Design review of the part built by this model. Coordinates are the model's own, in mm. A direction names the side the tool comes from. Give positions to 0.01 mm unless a question says otherwise; leave off trailing zeros. Order: outer loops, then holes, each group sorted by start corner. A loop starts at its lowest first (then second) coordinate and runs counter-clockwise, first axis right, second up.
```python
from build123d import *

# Parameters (mm, degrees)
SKETCH1_R           = 2.75
SKETCH1_R_2         = 15.875
SKETCH1_R_3         = 1.999996
BOSS_EXTRUDE1_DEPTH = 6.35
SKETCH2_R           = 2.6035
CUT_EXTRUDE1_DEPTH  = 6.35


with BuildPart() as part:
    # Sketch1 → Boss-Extrude1 (new body)
    with BuildSketch(Plane(origin=(0, 594.769027045, 0), x_dir=(1, 0, 0), z_dir=(0, 1, 0))):
        with BuildLine():
            Line((18.270000003, -51.148426992), (18.270000003, -71.640926991))
            Line((18.270000003, -71.640926991), (27.795000003, -71.640926991))
            Line((27.795000003, -71.640926991), (27.795000003, -19.656099647))
            ThreePointArc((27.795000003, -19.656099647), (28.316356539, -14.536226662), (29.859023577, -9.626533144))
            ThreePointArc((29.859023577, -9.626533144), (0, 35.706571509), (-29.859023577, -9.626533144))
            ThreePointArc((-29.859023577, -9.626533144), (-28.316356539, -14.536226662), (-27.795000003, -19.656099647))
            Line((-27.795000003, -19.656099647), (-27.795000003, -71.640926991))
            Line((-27.795000003, -71.640926991), (-18.270000003, -71.640926991))
            Line((-18.270000003, -71.640926991), (-18.270000003, -51.148426992))
            ThreePointArc((-18.270000003, -51.148426992), (-16.875096049, -47.780830946), (-13.507500003, -46.385926992))
            Line((-13.507500003, -46.385926992), (0, -46.385926991))
            Line((0, -46.385926991), (13.507500003, -46.385926992))
            ThreePointArc((13.507500003, -46.385926992), (16.875096049, -47.780830946), (18.270000003, -51.148426992))
        make_face()
        with Locations(Location((-23, -65.290926991, 0), (0, 0, 270))):
            Circle(SKETCH1_R, mode=Mode.SUBTRACT)
        with Locations(Location((-23, -47.290926991, 0), (0, 0, 270))):
            Circle(SKETCH1_R, mode=Mode.SUBTRACT)
        with Locations(Location((23, -47.290926991, 0), (0, 0, 270))):
            Circle(SKETCH1_R, mode=Mode.SUBTRACT)
        with Locations(Location((23, -65.290926991, 0), (0, 0, 270))):
            Circle(SKETCH1_R, mode=Mode.SUBTRACT)
        with Locations(Location((0, 3.206573009, 0), (0, 0, 270))):
            Circle(SKETCH1_R_2, mode=Mode.SUBTRACT)
        with Locations(Location((-15.697770542, -12.491197534, 0), (0, 0, 270))):
            Circle(SKETCH1_R_3, mode=Mode.SUBTRACT)
        with Locations(Location((-15.697770542, 18.904343551, 0), (0, 0, 270))):
            Circle(SKETCH1_R_3, mode=Mode.SUBTRACT)
        with Locations(Location((15.697770542, 18.904343551, 0), (0, 0, 270))):
            Circle(SKETCH1_R_3, mode=Mode.SUBTRACT)
        with Locations(Location((15.697770542, -12.491197534, 0), (0, 0, 270))):
            Circle(SKETCH1_R_3, mode=Mode.SUBTRACT)
    extrude(amount=BOSS_EXTRUDE1_DEPTH)

    # Sketch2 → Cut-Extrude1 (cut)
    with BuildSketch(Plane(origin=(0, 601.119027045, 0), x_dir=(1, 0, 0), z_dir=(0, 1, 0))):
        with Locations(Location((19.05, -23.780926991, 0), (0, 0, 270))):
            Circle(SKETCH2_R)
    extrude(amount=-CUT_EXTRUDE1_DEPTH, mode=Mode.SUBTRACT)


solid = part.part
```
1. Take a section at B-B (z = -18). State the section outline as (x, y) points, then the cut area to 3 significant figures.
Recorded:
outline: (-28.94, 594.77) - (-17.48, 594.77) - (-17.48, 601.12) - (-28.94, 601.12) - close; (-13.91, 594.77) - (-5.76, 594.77) - (-5.76, 601.12) - (-13.91, 601.12) - close; (5.76, 594.77) - (13.91, 594.77) - (13.91, 601.12) - (5.76, 601.12) - close; (17.48, 594.77) - (28.94, 594.77) - (28.94, 601.12) - (17.48, 601.12) - close
area: 249 mm2
2. For line 1 along X through (y, z) = (600, 56.5) (3 decimals); line 2 along X through (y, z) = (598.5, 23.5) (3 decimals); line 3 along Z through (x, y) = (25, 600), list the stretches that pass through material, from the lowest coordinate up.
Recorded:
line 1: x = -27.795 to -18.27, 18.27 to 27.795
line 2: x = -27.795 to 16.462, 21.638 to 27.795
line 3: z = -23.97 to 45.4, 49.18 to 63.4, 67.18 to 71.64
3. Machinability: for faces 1 (the face through (-16.912, 597.9, 47.818)), 2 (the face through (23.826, 597.9, 49.914)), 3 (the face through (-27.795, 598, 45)), which of the approach directions +Z, -Z, +X, -X, +Y, -Y give a long, thin tool a straight path to every point of the face, cutting with its end or side? Answer none if there is none.
Recorded:
face 1: +Z, +Y, -Y
face 2: +Y, -Y
face 3: +Z, -X, +Y, -Y
4. For pin 1 (6.5 mm diameter, centred on x = -15.7, z = 12.49, fed in from +Y); pin 2 (1 mm diameter, centred on x = 4.5, y = 599.5, fed in from -Z); pin 3 (1.5 mm diameter, centred on y = 595.5, z = 45.5, fed in from -X) (3 decimals); pin 4 (1.9 mm diameter, centred on x = -4, y = 596.5, fed in from +Z), all flat-tipped, find the tip position at first contact; note any pin that passes through.
Recorded:
pin 1: stops at y = 601.12
pin 2: stops at z = -35.46
pin 3: stops at x = -27.795
pin 4: stops at z = 46.39
5. Draft analysis for pull direction Z (two halves, no side actions). For faces 4 (the face through (-28.33, 597.9, 14.47)), 5 (the face through (18.27, 598, 61)), 6 (the face through (-6.08, 597.9, 11.46)), 7 (the face through (13.923, 597.9, -17.981)), state which applies: pulls with the +Z half, pulls with the -Z half, needs draft (parallel to the pull), parting line crosses it, or undercut.
Recorded:
face 4: pulls with the +Z half
face 5: needs draft
face 6: undercut
face 7: undercut
6. Take a section at A-A (z = 23). State the section outline as (x, y) points (3 decimals).
Recorded:
outline: (-27.795, 594.769) - (16.566, 594.769) - (16.566, 601.119) - (-27.795, 601.119) - close; (21.534, 594.769) - (27.795, 594.769) - (27.795, 601.119) - (21.534, 601.119) - close
7. Take a section at D-D (x = 23). State the section outline as (y, z) points.
Recorded:
outline: (594.77, -26.17) - (601.12, -26.17) - (601.12, 44.54) - (594.77, 44.54) - close; (594.77, 50.04) - (601.12, 50.04) - (601.12, 62.54) - (594.77, 62.54) - close; (594.77, 68.04) - (601.12, 68.04) - (601.12, 71.64) - (594.77, 71.64) - close
8. Take a section at C-C (y = 597.5). State how many separate pieces and enclosed holes the cut face has, then the cut area to 3 significant figures.
Recorded:
separate pieces: 1
enclosed holes: 10
area: 4,060 mm2
